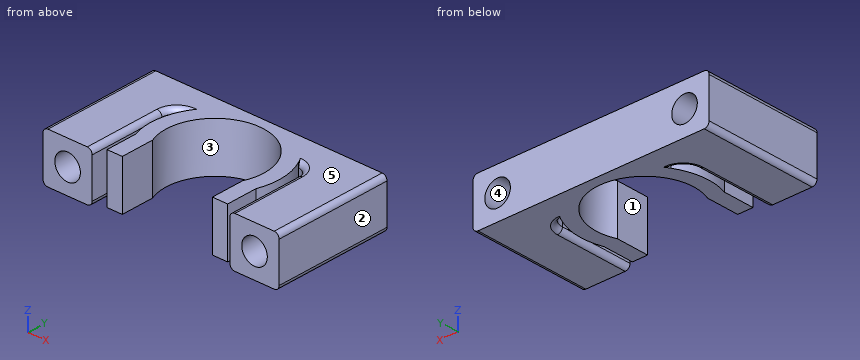
from build123d import *

# Parameters (mm, degrees)
BOSS_EXTRUDE1_DEPTH = 10
FILLET1_R           = 3
SKETCH2_R           = 2.6
CUT_EXTRUDE1_DEPTH  = 36.383612026
FILLET2_R           = 1


with BuildPart() as part:
    # Sketch1 → Boss-Extrude1 (new body)
    with BuildSketch(Plane.XY):
        with BuildLine():
            Line((-11.258330249, 6.5), (-14, 6.5))
            Line((-14, 6.5), (-14, -12))
            Line((-14, -12), (-24, -12))
            Line((-24, -12), (-24, 12))
            Line((-24, 12), (24, 12))
            Line((24, 12), (24, -12))
            Line((24, -12), (14, -12))
            Line((14, -12), (14, 6))
            Line((14, 6), (11.532562595, 6))
            ThreePointArc((11.532562595, 6), (12.967632791, 0.916787763), (12.262009764, -4.317767543))
            Line((12.262009764, -4.317767543), (12.262009764, -7.605344152))
            Line((12.262009764, -7.605344152), (12.262009764, -10.605344152))
            Line((12.262009764, -10.605344152), (9.157960199, -10.605344152))
            Line((9.157960199, -10.605344152), (9.157960199, -3.890278267))
            ThreePointArc((9.157960199, -3.890278267), (0, 9.95), (-9.157960199, -3.890278267))
            Line((-9.157960199, -3.890278267), (-9.157960199, -10.605344152))
            Line((-9.157960199, -10.605344152), (-12.262862833, -10.605344152))
            Line((-12.262862833, -10.605344152), (-12.262862833, -7.605344152))
            Line((-12.262862833, -7.605344152), (-12.262862833, -4.315344152))
            ThreePointArc((-12.262862833, -4.315344152), (-12.944286318, 1.202269405), (-11.258330249, 6.5))
        make_face()
    extrude(amount=BOSS_EXTRUDE1_DEPTH)

    # Fillet1
    # the kernel refuses this fillet: 3 mm, written as the material it adds along each edge
    with BuildSketch(Plane(origin=(14, 6, 0), x_dir=(-1, 0, 0), z_dir=(0, 0, 1))) as fillet1_piece_1:
        with BuildLine():
            CenterArc((3, 2.952351111), FILLET1_R, 180, 79.774609626)
            Line((0, 2.952351111), (-0.06, 2.952351111))
            Line((-0.06, 2.952351111), (-0.06, 0))
            Line((-0.06, 0), (0, -0.06))
            ThreePointArc((0, -0.06), (1.233718703, -0.06), (2.456786153, -0.059047022))
            Line((2.456786153, -0.059047022), (2.467437405, 0))
        make_face()
    extrude(amount=10)
    with BuildSketch(Plane(origin=(-14, 6.5, 0), x_dir=(1, 0, 0), z_dir=(0, 0, 1))) as fillet1_piece_2:
        with BuildLine():
            CenterArc((3, -2.988856886), FILLET1_R, 94.93986201, 85.06013799)
            Line((0, -2.988856886), (-0.06, -2.988856886))
            Line((-0.06, -2.988856886), (-0.06, 0))
            Line((-0.06, 0), (0, 0.06))
            ThreePointArc((0, 0.06), (1.370834875, 0.06), (2.736503146, 0.059777138))
            Line((2.736503146, 0.059777138), (2.741669751, 0))
        make_face()
    extrude(amount=10)

    # Sketch2 → Cut-Extrude1 (cut, through all)
    with BuildSketch(Plane.XZ.offset(12)):
        with Locations(Location((-19, 5, 0), (0, 0, 270))):
            Circle(SKETCH2_R)
        with Locations(Location((19, 5, 0), (0, 0, 270))):
            Circle(SKETCH2_R)
    extrude(amount=-CUT_EXTRUDE1_DEPTH, mode=Mode.SUBTRACT)

    # Fillet2
    # the kernel refuses this fillet: 1 mm, written as the material it takes off along each edge
    with BuildSketch(Plane(origin=(-24, -14.5, 0), x_dir=(1, 0, 0), z_dir=(0, 1, 0)), Plane(origin=(24, 14.5, 0), x_dir=(-1, 0, 0), z_dir=(0, -1, 0))) as fillet2_piece_1:
        with BuildLine():
            CenterArc((FILLET2_R, -FILLET2_R), FILLET2_R, 90, 90)
            Line((0, -FILLET2_R), (0, 0))
            Line((0, 0), (FILLET2_R, 0))
        make_face()
    extrude(amount=29, mode=Mode.SUBTRACT)
    with BuildSketch(Plane(origin=(14, -14.5, 0), x_dir=(1, 0, 0), z_dir=(0, 1, 0))) as fillet2_piece_2:
        with BuildLine():
            CenterArc((FILLET2_R, -FILLET2_R), FILLET2_R, 90, 90)
            Line((0, -FILLET2_R), (0, 0))
            Line((0, 0), (FILLET2_R, 0))
        make_face()
    extrude(amount=17.547648889, mode=Mode.SUBTRACT)
    with BuildSketch(Plane(origin=(14, -14.5, 10), x_dir=(1, 0, 0), z_dir=(0, 1, 0))) as fillet2_piece_3:
        with BuildLine():
            CenterArc((FILLET2_R, FILLET2_R), FILLET2_R, 180, 90)
            Line((0, FILLET2_R), (0, 0))
            Line((0, 0), (FILLET2_R, 0))
        make_face()
    extrude(amount=17.547648889, mode=Mode.SUBTRACT)
    with BuildSketch(Plane(origin=(-14, 3.511143114, 0), x_dir=(0, 0, 1), z_dir=(0, -1, 0))) as fillet2_piece_4:
        with BuildLine():
            CenterArc((FILLET2_R, FILLET2_R), FILLET2_R, 180, 90)
            Line((0, FILLET2_R), (0, 0))
            Line((0, 0), (FILLET2_R, 0))
        make_face()
    extrude(amount=18.011143114, mode=Mode.SUBTRACT)
    with BuildSketch(Plane(origin=(-14, 3.511143114, 10), x_dir=(0, 0, -1), z_dir=(0, -1, 0))) as fillet2_piece_5:
        with BuildLine():
            CenterArc((FILLET2_R, -FILLET2_R), FILLET2_R, 90, 90)
            Line((0, -FILLET2_R), (0, 0))
            Line((0, 0), (FILLET2_R, 0))
        make_face()
    extrude(amount=18.011143114, mode=Mode.SUBTRACT)
    with BuildSketch(Plane(origin=(11, 3.047648889, 0), x_dir=(1, 0, 0), z_dir=(0, -1, 0))) as fillet2_piece_6_section:
        with BuildLine():
            CenterArc((3 + FILLET2_R, FILLET2_R), FILLET2_R, 180, 90)
            Line((3, FILLET2_R), (3, 0))
            Line((3, 0), (3 + FILLET2_R, 0))
        make_face()
    fillet2_piece_6 = revolve(axis=Axis((11, 3.047648889, 0), (0, 0, 1)), revolution_arc=127.536161061, mode=Mode.PRIVATE)
    fillet2_piece_6 = fillet2_piece_6 - Plane(origin=(0, 0, 0.285399127), x_dir=(0.8871201995900612, 0.46153846153846184, 0), z_dir=(0, 0, -1)) * Cylinder(13, 16, mode=Mode.PRIVATE)
    add(fillet2_piece_6, mode=Mode.SUBTRACT)
    with BuildSketch(Plane(origin=(11, 3.047648889, 10), x_dir=(1, 0, 0), z_dir=(0, -1, 0))) as fillet2_piece_7_section:
        with BuildLine():
            CenterArc((3 + FILLET2_R, -FILLET2_R), FILLET2_R, 90, 90)
            Line((3, -FILLET2_R), (3, 0))
            Line((3, 0), (3 + FILLET2_R, 0))
        make_face()
    fillet2_piece_7 = revolve(axis=Axis((11, 3.047648889, 10), (0, 0, 1)), revolution_arc=127.536161061, mode=Mode.PRIVATE)
    fillet2_piece_7 = fillet2_piece_7 - Plane(origin=(0, 0, 9.714600873), x_dir=(0.8871201995900612, 0.46153846153846184, 0), z_dir=(0, 0, -1)) * Cylinder(13, 16, mode=Mode.PRIVATE)
    add(fillet2_piece_7, mode=Mode.SUBTRACT)
    with BuildSketch(Plane(origin=(-11, 3.511143114, 0), x_dir=(0.6797454248064234, 0.7334481286735518, 0), z_dir=(0.7334481286735518, -0.6797454248064234, 0))) as fillet2_piece_8_section:
        with BuildLine():
            CenterArc((3 + FILLET2_R, FILLET2_R), FILLET2_R, 180, 90)
            Line((3 + FILLET2_R, 0), (3, 0))
            Line((3, 0), (3, FILLET2_R))
        make_face()
    fillet2_piece_8 = revolve(axis=Axis((-11, 3.511143114, 0), (0, 0, 1)), revolution_arc=132.823752842, mode=Mode.PRIVATE)
    fillet2_piece_8 = fillet2_piece_8 - Plane(origin=(0, 0, 0.285251349), x_dir=(-0.9432971409738413, -0.3319495501285957, 0), z_dir=(0, 0, -1)) * Cylinder(13, 17, mode=Mode.PRIVATE)
    add(fillet2_piece_8, mode=Mode.SUBTRACT)
    with BuildSketch(Plane(origin=(-11, 3.511143114, 10), x_dir=(0.6797454248064234, 0.7334481286735518, 0), z_dir=(0.7334481286735518, -0.6797454248064234, 0))) as fillet2_piece_9_section:
        with BuildLine():
            CenterArc((3 + FILLET2_R, -FILLET2_R), FILLET2_R, 90, 90)
            Line((3 + FILLET2_R, 0), (3, 0))
            Line((3, 0), (3, -FILLET2_R))
        make_face()
    fillet2_piece_9 = revolve(axis=Axis((-11, 3.511143114, 10), (0, 0, 1)), revolution_arc=132.823752842, mode=Mode.PRIVATE)
    fillet2_piece_9 = fillet2_piece_9 - Plane(origin=(0, 0, 9.714748651), x_dir=(-0.9432971409738413, -0.3319495501285957, 0), z_dir=(0, 0, -1)) * Cylinder(13, 17, mode=Mode.PRIVATE)
    add(fillet2_piece_9, mode=Mode.SUBTRACT)
    with BuildSketch(Plane(origin=(24, 14.5, 10), x_dir=(-1, 0, 0), z_dir=(0, -1, 0)), Plane(origin=(-24, -14.5, 10), x_dir=(1, 0, 0), z_dir=(0, 1, 0))) as fillet2_piece_10:
        with BuildLine():
            CenterArc((FILLET2_R, FILLET2_R), FILLET2_R, 180, 90)
            Line((0, FILLET2_R), (0, 0))
            Line((0, 0), (FILLET2_R, 0))
        make_face()
    extrude(amount=29, mode=Mode.SUBTRACT)


solid = part.part
Here's how the part is built. I have some questions about the finished solid (model axes, mm). Face numbers are marked on the shaded views. A direction names the side the tool comes from. Coordinates: 2 decimals unless noted, no trailing zeros. Loops run counter-clockwise (first coordinate to the right, second up) from the corner with the lowest first, then second, coordinate; pieces in that order, holes last. Notation, with made-up numbers: (52.5, -20) -> (105.5, -20) arc R17 cw to (105.5, -12) -> close; hole circle Ø10 at (15.25, 43.25). An arc over 180 degrees is marked (long way). Use one line per item in the form item = value. Start each with the question number.
(1) If we section it at B-B (x = -19): Please give me the cut outline in (y, z), then the cut area to 3 significant figures.
(2) Please list where these lines run through material, in increasing order: line 1 along X through (y, z) = (-6, 5); line 2 along X through (y, z) = (-9.25, 0.75); line 3 along X through (y, z) = (-10.75, 6).
(3) Will these pins go through, and if not, where does the flat tip stop? pin 1 (2 mm diameter, centred on x = -19, z = 5.5, fed in from +Y); pin 2 (6 mm diameter, centred on x = -8, z = 6, fed in from -Y).
(4) On a 3-axis mill with a long thin cutter (end or side, diameter ignored), from which of +Z, -Z, +X, -X, +Y, -Y can I reach the whole of each face in a straight line? I mean the marked faces 1 and 2. Say none if no direction works.
(5) If we section it at A-A (y = 0): Please give me the cut outline in (x, z).
(6) If we section it at C-C (z = 8.5): Please give me the cut outline in (x, y).
(7) We'd pull the mould along Z, two halves only. Please class the marked faces 3, 4 and 5: pulls with the +Z half, pulls with the -Z half, needs draft (parallel to the pull), parting line crosses it, or undercut.
(8) If we section it at D-D (z = 4.75): Please give me the cut outline in (x, y), then the cut area to 3 significant figures.
Verdict:
q1.outline = (-12, 0) -> (12, 0) -> (12, 2.4) -> (-12, 2.4) -> close; (-12, 7.6) -> (12, 7.6) -> (12, 10) -> (-12, 10) -> close
q1.area = 115 mm²
q2.line_1 = -24 to -21.6, -16.4 to -14, -12.26 to -9.16, 9.16 to 12.26, 14 to 16.4, 21.6 to 24
q2.line_2 = -23.97 to -14.03, -12.26 to -9.16, 9.16 to 12.26, 14.03 to 23.97
q2.line_3 = -24 to -21.4, -16.6 to -14, 14 to 16.6, 21.4 to 24
q3.pin_1 = through
q3.pin_2 = -10.61
q4.face_1 = +Z, -Z, -Y
q4.face_2 = +Z, -Z, +X, +Y, -Y
q5.outline = (-24, 1) arc R1 ccw to (-23, 0) -> (-15, 0) arc R1 ccw to (-14, 1) -> (-14, 9) arc R1 ccw to (-15, 10) -> (-23, 10) arc R1 ccw to (-24, 9) -> close; (-13, 0) -> (-9.95, 0) -> (-9.95, 10) -> (-13, 10) -> close; (9.95, 0) -> (13, 0) -> (13, 10) -> (9.95, 10) -> close; (14, 1) arc R1 ccw to (15, 0) -> (23, 0) arc R1 ccw to (24, 1) -> (24, 9) arc R1 ccw to (23, 10) -> (15, 10) arc R1 ccw to (14, 9) -> close; hole circle Ø5.2 at (-19, 5); hole circle Ø5.2 at (19, 5)
q6.outline = (-24, -12) -> (-14, -12) -> (-14, 3.51) arc R3 cw to (-11.26, 6.5) arc R13 ccw to (-12.26, -4.32) -> (-12.26, -10.61) -> (-9.16, -10.61) -> (-9.16, -3.89) arc R9.95 cw (long way) to (9.16, -3.89) -> (9.16, -10.61) -> (12.26, -10.61) -> (12.26, -4.32) arc R13 ccw to (11.53, 6) arc R3 cw to (14, 3.05) -> (14, -12) -> (24, -12) -> (24, 12) -> (-24, 12) -> close
q7.face_3 = needs draft
q7.face_4 = undercut
q7.face_5 = pulls with the +Z half
q8.outline = (-24, -12) -> (-21.59, -12) -> (-21.59, 12) -> (-24, 12) -> close; (-16.41, -12) -> (-14, -12) -> (-14, 3.51) arc R3 cw to (-11.26, 6.5) arc R13 ccw to (-12.26, -4.32) -> (-12.26, -10.61) -> (-9.16, -10.61) -> (-9.16, -3.89) arc R9.95 cw (long way) to (9.16, -3.89) -> (9.16, -10.61) -> (12.26, -10.61) -> (12.26, -4.32) arc R13 ccw to (11.53, 6) arc R3 cw to (14, 3.05) -> (14, -12) -> (16.41, -12) -> (16.41, 12) -> (-16.41, 12) -> close; (21.59, -12) -> (24, -12) -> (24, 12) -> (21.59, 12) -> close
q8.area = 463 mm²
